Autodesk Inventor part; units mm, degrees
ref_plane "YZ Plane" through (0, 0, 0) normal (1, 0, 0) x (0, 1, 0)
ref_plane "XZ Plane" through (0, 0, 0) normal (0, 1, 0) x (-1, 0, 0)
ref_plane "XY Plane" through (0, 0, 0) normal (0, 0, 1) x (1, 0, 0)
sketch "Sketch1" plane through (0, 0, 0) normal (0, 0, 1) x (1, 0, 0)
  circle A0 centre (0, 0) radius 1.7526
  dimension "d0" = 3.5052
extrude "Extrusion1" add sketch "Sketch1" along normal blind 12.7
sketch "Sketch2" plane through (0, 0, 0) normal (0, 0, -1) x (-1, 0, 0)
  circle A0 centre (0, 0) radius 1.7526 construction
  circle A1 centre (0, 0) radius 2.8702
  dimension "d3" = 5.7404
extrude "Extrusion2" add sketch "Sketch2" along normal blind 3.5052
sketch "Sketch3" plane through (0, 0, -3.5052) normal (0, 0, -1) x (-1, 0, 0)
  circle A0 centre (0, 0) radius 2.8702
  line L0 (0, 1.604) -> (1.3891, 0.802)
  line L1 (1.3891, 0.802) -> (1.3891, -0.802)
  line L2 (1.3891, -0.802) -> (0, -1.604)
  line L3 (0, -1.604) -> (-1.3891, -0.802)
  line L4 (-1.3891, -0.802) -> (-1.3891, 0.802)
  line L5 (-1.3891, 0.802) -> (0, 1.604)
  dimension "d6" = 2.7781
extrude "Extrusion3" cut sketch "Sketch3" against normal blind 1.7526 contours L0 L1 L2 L3 L4 L5
thread "Thread1"
chamfer "Chamfer1" distance 0.508 angle 45 1 edges at (-1.7526, 0, 12.7)
properties part number "6-32 SHCS x500" material "Stainless Steel"
Check sheet for the modelled part. Datum: model origin and axes. Units: mm. A direction names the side the tool comes from. Give positions to 0.01 mm unless a question says otherwise; leave off trailing zeros. Write each loop counter-clockwise with the first axis right and the second up, starting at its lowest first coordinate (ties: lowest second). Pieces come first, ordered by that corner, then holes. Notation, with made-up numbers: (-18, 8.25) -> (19, 8.25) arc R16 cw to (19, 33.25) -> close; hole circle Ø2 at (16.5, 61). An arc over 180 degrees is marked (long way). One line per item, written item: value. Start each with the question number.
Item 1: Section check C-C on x = 2.35. Record the cut outline in (y, z), then the cut area to 3 significant figures.
Item 2: Section check A-A on y = 0. Record the cut outline in (x, z).
Item 3: Draft check along Y on faces 4 (the flat face through (-0.7, -1.2, -2.6)), 5 (the flat face through (0, 0, 12.7)), 6 (the cylindrical face through (2.278, 1.746, -1.728)). Enter one of: +Y half, -Y half, draft (parallel to the pull), parting line (faces both ways), or undercut.
Item 4: Gauge pin test, flat ends, axial feed: pin 1 (1.5 mm diameter, centred on x = -1.5, z = 4, fed in from +Y); pin 2 (2 mm diameter, centred on x = -1.5, y = 0, fed in from +Z); pin 3 (1.5 mm diameter, centred on y = -1.5, z = 10, fed in from +X). Record the tip position at first contact, or that the pin passes through.
Item 5: Material ranges on probe 1 along Y at (x, z) = (0.1, 2.25); probe 2 along Z at (x, y) = (-1.9, 2.1); probe 3 along Z at (x, y) = (0.05, 0), recorded low to high. Write a range as from..to.
Item 6: Section check D-D on z = 1.5. Record the cut outline in (x, y).
Item 7: Section check B-B on z = -0.25. Record the cut outline in (x, y).
Item 8: Tool access check on faces 1 (the flat face through (0, -2, 0)), 2 (the flat face through (-1.2, -1.2, -3.505)), 3 (the flat face through (1.389, 0, -3)). Record the directions out of +Z, -Z, +X, -X, +Y, -Y that give a thin tool (end or side, any length) a straight path to the whole face; none if there is none.
Results list:
1. outline: (-1.65, -3.51) -> (1.65, -3.51) -> (1.65, 0) -> (-1.65, 0) -> close
1. area: 11.6 mm²
2. outline: (-2.87, -3.51) -> (-1.39, -3.51) -> (-1.39, -1.75) -> (1.39, -1.75) -> (1.39, -3.51) -> (2.87, -3.51) -> (2.87, 0) -> (1.75, 0) -> (1.75, 12.19) -> (1.24, 12.7) -> (-1.24, 12.7) -> (-1.75, 12.19) -> (-1.75, 0) -> (-2.87, 0) -> close
3. face 4: undercut
3. face 5: draft
3. face 6: parting line
4. pin 1: y = 1.58
4. pin 2: z = 12.7
4. pin 3: x = 1.58
5. probe 1: -1.75..1.75
5. probe 2: -3.51..0
5. probe 3: -1.75..12.7
6. outline: circle Ø3.51 at (0, 0)
7. outline: circle Ø5.74 at (0, 0)
8. face 1: +Z
8. face 2: -Z, +X, -X, +Y, -Y
8. face 3: -Z
